Answer from the drawing. Dimensions are ordinates in mm from the lowest x, y and z of the part. Coordinates: 2 decimals unless noted, no trailing zeros. Write each loop counter-clockwise with the first axis right and the second up, starting at its lowest first coordinate (ties: lowest second). Pieces come first, ordered by that corner, then holes.
1) Find the intervals of material crossed by line 1 (X direction, y = 3.75, z = 20); line 2 (X direction, y = 6.5, z = 22); line 3 (X direction, y = 4, z = 9.5), in increasing order.
2) The part is cut by section B-B (z = 37). Determine the outline of the cut face in (x, y).
3) Each of these flat-tipped pins is pushed along its axis until it touches: pin 1 Ø5.5 at (x, z) = (7.5, 19) entering from +Y; pin 2 Ø3 at (x, y) = (57, 4) entering from -Z; pin 3 Ø2 at (y, z) = (3.5, 6.5) entering from -X; pin 4 Ø12 at (x, z) = (24.5, 18.5) entering from +Y. Where does it stop, or does it pass through?
4) Determine the mould class of the marked faces 1, 2, 3 and 4 for opening direction X: +X half, -X half, draft (parallel to the pull), parting line (faces both ways), or undercut.
5) The part is cut by section D-D (x = 40). Determine the outline of the cut face in (y, z).
6) The part is cut by section A-A (y = 3). Determine the outline of the cut face in (x, z), then the cut area to 3 significant figures.
7) The part is cut by section C-C (x = 59). Determine the outline of the cut face in (y, z), then the cut area to 3 significant figures.
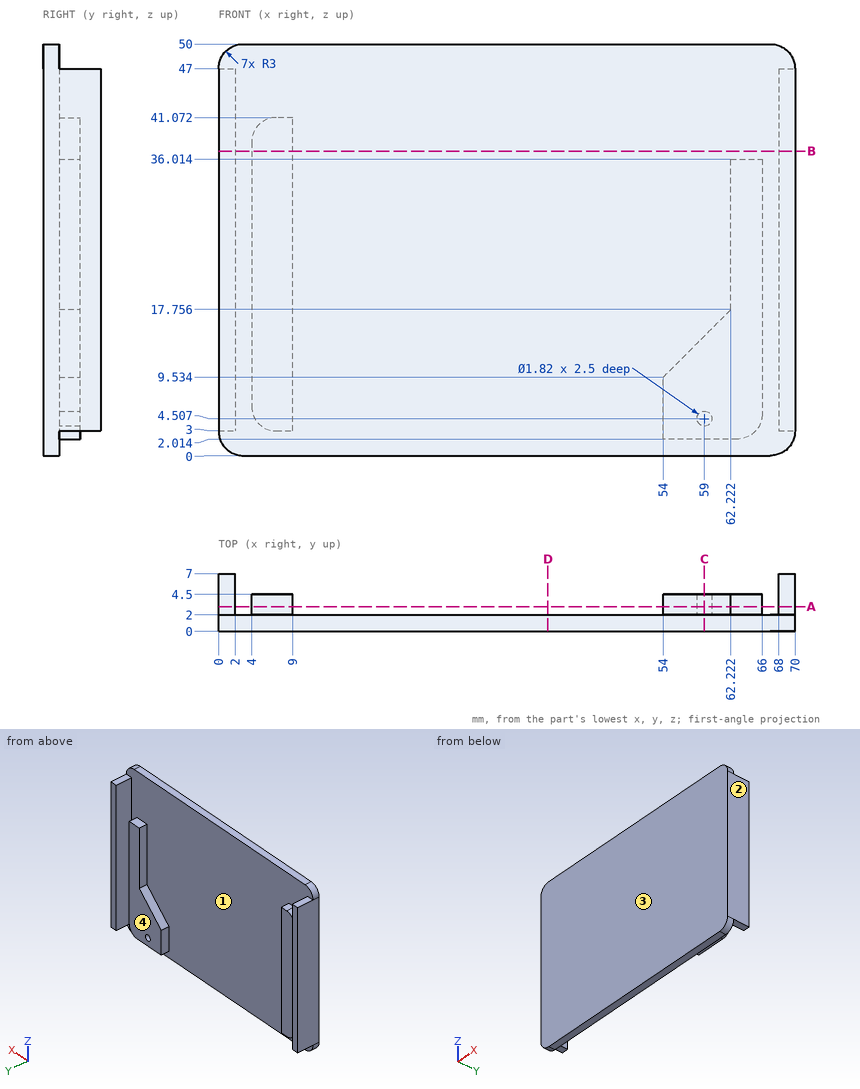
Reported:
1. line 1: x = 0 to 2, 4 to 9, 62.22 to 66, 68 to 70
1. line 2: x = 0 to 2, 68 to 70
1. line 3: x = 0 to 2, 4 to 9, 54 to 66, 68 to 70
2. outline: (0, 0) - (70, 0) - (70, 7) - (68, 7) - (68, 2) - (9, 2) - (9, 4.5) - (4, 4.5) - (4, 2) - (2, 2) - (2, 7) - (0, 7) - close
3. pin 1: stops at y = 4.5
3. pin 2: stops at z = 2.01
3. pin 3: stops at x = 0
3. pin 4: stops at y = 2
4. face 1: undercut
4. face 2: +X half
4. face 3: draft
4. face 4: undercut
5. outline: (0, 0) - (2, 0) - (2, 50) - (0, 50) - close
6. outline: (0, 3) - (2, 3) - (2, 47) - (0, 47) - close; (4, 6) arc R3 ccw to (7, 3) - (9, 3) - (9, 41.07) - (7, 41.07) arc R3 ccw to (4, 38.07) - close; (54, 2.01) - (63, 2.01) arc R3 ccw to (66, 5.01) - (66, 36.01) - (62.22, 36.01) - (62.22, 17.76) - (54, 9.53) - close; (68, 3) - (70, 3) - (70, 47) - (68, 47) - close; hole circle Ø1.82 at (59, 4.51)
6. area: 582 mm2
7. outline: (0, 0) - (2, 0) - (2, 2.01) - (4.5, 2.01) - (4.5, 3.6) - (2, 3.6) - (2, 5.42) - (4.5, 5.42) - (4.5, 14.53) - (2, 14.53) - (2, 50) - (0, 50) - close
7. area: 127 mm2
